The listing builds one solid part. Answer for the finished solid, in the listing's coordinates (mm). Face numbers are marked on the shaded views. A direction names the side the tool comes from. Coordinates: 2 decimals unless noted, no trailing zeros. Loops run counter-clockwise (first coordinate to the right, second up) from the corner with the lowest first, then second, coordinate; pieces in that order, holes last. Notation, with made-up numbers: M 4.5,40.5 L 27.5,40.5 A22 cw 27.5,55.5 Z; hole C 12.5,-6 d2. An arc over 180 degrees is marked long. Answer as CSV lines item,"result". Start each with the question number.
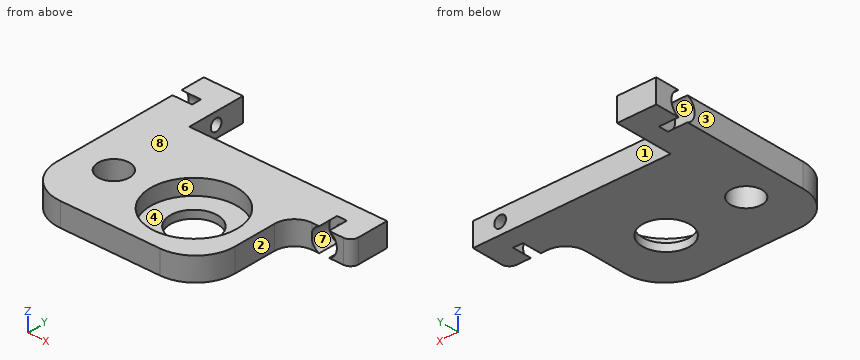
```python
from build123d import *

# Parameters (mm, degrees)
CROQUIS1_R              = 4
CROQUIS1_R_2            = 6
SALIENTE_EXTRUIR2_DEPTH = 6
CROQUIS2_R              = 11
CORTAR_EXTRUIR1_DEPTH   = 4
CROQUIS3_R              = 1.5
CORTAR_EXTRUIR2_DEPTH   = 71.672536391
CROQUIS4_R              = 1.5
CORTAR_EXTRUIR3_DEPTH   = 63.337848856
CROQUIS5_R              = 3.25
CORTAR_EXTRUIR4_DEPTH   = 5
CROQUIS6_R              = 3.25
CORTAR_EXTRUIR5_DEPTH   = 5


with BuildPart() as part:
    # Croquis1 → Saliente-Extruir2 (new body)
    with BuildSketch(Plane.XY):
        with BuildLine():
            Line((-50.43, 0), (0, 0))
            Line((0, 0), (0, -8))
            ThreePointArc((0, -8), (-0.585786438, -9.414213562), (-2, -10))
            Line((-2, -10), (-10, -10))
            ThreePointArc((-10, -10), (-13.535533906, -11.464466094), (-15, -15))
            Line((-15, -15), (-15, -26.15))
            ThreePointArc((-15, -26.15), (-17.928932188, -33.221067812), (-25, -36.15))
            Line((-25, -36.15), (-50.43, -36.15))
            ThreePointArc((-50.43, -36.15), (-57.501067812, -33.221067812), (-60.43, -26.15))
            Line((-60.43, -26.15), (-60.43, 15))
            Line((-60.43, 15), (-50.43, 15))
            Line((-50.43, 15), (-50.43, 0))
        make_face()
        with Locations((-50.43, -21.15)):
            Circle(CROQUIS1_R, mode=Mode.SUBTRACT)
        with Locations((-30, -21.15)):
            Circle(CROQUIS1_R_2, mode=Mode.SUBTRACT)
    extrude(amount=SALIENTE_EXTRUIR2_DEPTH)

    # Croquis2 → Cortar-Extruir1 (cut)
    with BuildSketch(Plane.XY.offset(6)):
        with Locations((-30, -21.15)):
            Circle(CROQUIS2_R)
    extrude(amount=-CORTAR_EXTRUIR1_DEPTH, mode=Mode.SUBTRACT)

    # Croquis3 → Cortar-Extruir2 (cut, through all)
    with BuildSketch(Plane(origin=(0, 0, 0), x_dir=(-1, 0, 0), z_dir=(0, 1, 0))):
        with Locations(Location((6.93, 3, 0), (0, 0, 90))):
            Circle(CROQUIS3_R)
    extrude(amount=-CORTAR_EXTRUIR2_DEPTH, mode=Mode.SUBTRACT)

    # Croquis4 → Cortar-Extruir3 (cut, through all)
    with BuildSketch(Plane(origin=(-50.43, 0, 0), x_dir=(0, 0, -1), z_dir=(1, 0, 0))):
        with Locations((-3, 7.5)):
            Circle(CROQUIS4_R)
    extrude(amount=-CORTAR_EXTRUIR3_DEPTH, mode=Mode.SUBTRACT)

    # Croquis5 → Cortar-Extruir4 (cut)
    with BuildSketch(Plane.ZY.offset(60.43)):
        with Locations((3, 7.5)):
            Circle(CROQUIS5_R)
    extrude(amount=-CORTAR_EXTRUIR4_DEPTH, mode=Mode.SUBTRACT)

    # Croquis6 → Cortar-Extruir5 (cut)
    with BuildSketch(Plane.XZ.offset(10)):
        with Locations((-6.93, 3)):
            Circle(CROQUIS6_R)
    extrude(amount=-CORTAR_EXTRUIR5_DEPTH, mode=Mode.SUBTRACT)


solid = part.part
```
Item 1: Consider line 1 (Y direction, x = -30, z = 4.25); line 2 (Y direction, x = -30, z = 0.7); line 3 (X direction, y = -1.4, z = 3). Determine where each line is inside the solid, lowest interval first.
Item 2: Section B-B on x = -6.93 is taken. Determine the outline of the cut face in (y, z).
Item 3: Section C-C on y = -21.15 is taken. Determine the outline of the cut face in (x, z), then the cut area to 3 significant figures.
Item 4: Section D-D on y = 7.5 is taken. Determine the outline of the cut face in (x, z).
Item 5: For the marked faces 1, 2, 3, 4 and 5, determine the directions among +Z, -Z, +X, -X, +Y, -Y from which every point of the face is accessible in a straight line to the end or side of a thin tool.
Item 6: Each of these flat-tipped pins is pushed along its axis until it touches: P1, Ø2, axis at x = -9, z = 1, coming from the -Y side; P2, Ø6.5, axis at x = -26.5, y = -25.5, coming from the +Z side; P3, Ø3, axis at x = -7, z = 4, coming from the -Y side. Where does it stop, or does it pass through?
Item 7: For a pull along Z with two mould halves and no side action, classify the marked faces 6, 7 and 8 as pulls with the +Z half, pulls with the -Z half, needs draft (parallel to the pull), parting line crosses it, or undercut.
Item 8: Section A-A on z = 3 is taken. State how many separate pieces and enclosed holes the cut face has, then the cut area to 3 significant figures.
Results are:
1,line 1,"-36.15 to -32.15, -10.15 to 0"
1,line 2,"-36.15 to -27.15, -15.15 to 0"
1,line 3,"-60.43 to -8.43, -5.43 to 0"
2,outline,"M -5,0 L 0,0 L 0,1.5 L -5,1.5 Z; M -5,4.5 L 0,4.5 L 0,6 L -5,6 Z"
3,outline,"M -60.43,0 L -54.43,0 L -54.43,6 L -60.43,6 Z; M -46.43,0 L -36,0 L -36,2 L -41,2 L -41,6 L -46.43,6 Z; M -24,0 L -15,0 L -15,6 L -19,6 L -19,2 L -24,2 Z"
3,area,"113 mm²"
4,outline,"M -55.43,0 L -50.43,0 L -50.43,1.5 L -55.43,1.5 Z; M -55.43,4.5 L -50.43,4.5 L -50.43,6 L -55.43,6 Z"
5,face 1,"+Z, -Z, +X, +Y"
5,face 2,"+Z, -Z, +X, -Y"
5,face 3,"+Z, -Z, -X, +Y, -Y"
5,face 4,"+Z"
5,face 5,"-X"
6,P1,"y = -10"
6,P2,"z = 2"
6,P3,"y = -5"
7,face 6,"needs draft"
7,face 7,"undercut"
7,face 8,"pulls with the +Z half"
8,separate pieces,"3"
8,enclosed holes,"2"
8,area,"1,380 mm²"
